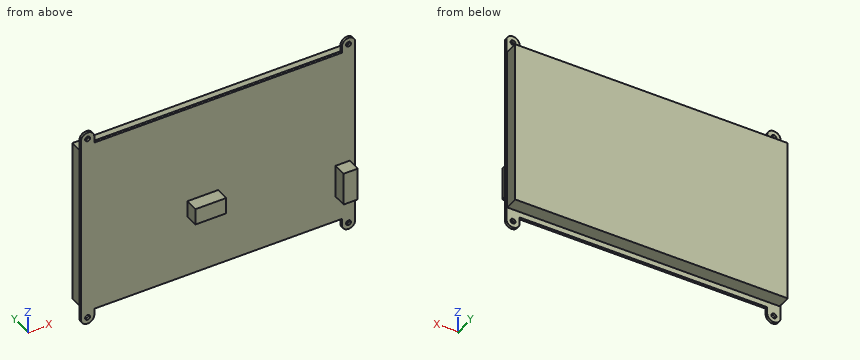
```python
from build123d import *

# Parameters (mm, degrees)
SKETCH1_R           = 1.5
BOSS_EXTRUDE1_DEPTH = 1.5
SKETCH2_W           = 8.49594542
SKETCH2_H           = 19.836738538
SKETCH2_W_2         = 18.514132699
SKETCH2_H_2         = 9.878260544
BOSS_EXTRUDE2_DEPTH = 8
SKETCH3_W           = 164
SKETCH3_H           = 100
BOSS_EXTRUDE3_DEPTH = 8


with BuildPart() as part:
    # Sketch1 → Boss-Extrude1 (new body)
    with BuildSketch(Plane(origin=(0, 0, 0), x_dir=(1, 0, 0), z_dir=(0, 1, 0))):
        with BuildLine():
            Line((-74.5, -53.5), (74.5, -53.5))
            Line((74.5, -53.5), (74.5, -57.5))
            ThreePointArc((74.5, -57.5), (78.5, -61.5), (82.5, -57.5))
            Line((82.5, -57.5), (82.5, -23.877612559))
            Line((82.5, -23.877612559), (82.5, 23.877612559))
            Line((82.5, 23.877612559), (82.5, 57.5))
            ThreePointArc((82.5, 57.5), (78.5, 61.5), (74.5, 57.5))
            Line((74.5, 57.5), (74.5, 53.5))
            Line((74.5, 53.5), (-74.5, 53.5))
            Line((-74.5, 53.5), (-74.5, 57.5))
            ThreePointArc((-74.5, 57.5), (-78.5, 61.5), (-82.5, 57.5))
            Line((-82.5, 57.5), (-82.5, 23.877612559))
            Line((-82.5, 23.877612559), (-82.5, -23.877612559))
            Line((-82.5, -23.877612559), (-82.5, -57.5))
            ThreePointArc((-82.5, -57.5), (-78.5, -61.5), (-74.5, -57.5))
            Line((-74.5, -57.5), (-74.5, -53.5))
        make_face()
        with Locations(Location((78.5, 57.5, 0), (0, 0, 270))):
            Circle(SKETCH1_R, mode=Mode.SUBTRACT)
        with Locations(Location((-78.5, 57.5, 0), (0, 0, 90))):
            Circle(SKETCH1_R, mode=Mode.SUBTRACT)
        with Locations(Location((78.5, -57.5, 0), (0, 0, 90))):
            Circle(SKETCH1_R, mode=Mode.SUBTRACT)
        with Locations(Location((-78.5, -57.5, 0), (0, 0, 270))):
            Circle(SKETCH1_R, mode=Mode.SUBTRACT)
    extrude(amount=BOSS_EXTRUDE1_DEPTH)

    # Sketch2 → Boss-Extrude2 (add)
    with BuildSketch(Plane.XZ):
        with Locations((74.922222093, -27.720858346)):
            Rectangle(SKETCH2_W, SKETCH2_H)
        with Locations((-9.25706635, -10.936720321)):
            Rectangle(SKETCH2_W_2, SKETCH2_H_2)
    extrude(amount=BOSS_EXTRUDE2_DEPTH)

    # Sketch3 → Boss-Extrude3 (add)
    with BuildSketch(Plane(origin=(0, 1.5, 0), x_dir=(1, 0, 0), z_dir=(0, 1, 0))):
        Rectangle(SKETCH3_W, SKETCH3_H)
    extrude(amount=BOSS_EXTRUDE3_DEPTH)


solid = part.part
```
The listing builds one solid part. Answer for the finished solid, in the listing's coordinates (mm). Round coordinates to 2 decimals unless told otherwise and drop trailing zeros. Order: outer loops, then holes, each group sorted by start corner. A loop starts at its lowest first (then second) coordinate and runs counter-clockwise, first axis right, second up. Notation, with made-up numbers: (47.25, -22.5) -> (88.25, -22.5) arc R16 ccw to (88.25, -9.5) -> close; hole circle Ø5 at (39, 86). An arc over 180 degrees is marked (long way). Answer as CSV lines item,"result". Start each with the question number.
(1) Flat-ended cylindrical pins translate along their axes: pin 1 Ø1 at (y, z) = (-2, 39) entering from +X (1 decimal); pin 2 Ø3 at (x, z) = (6, -47) entering from -Y; pin 3 Ø5 at (x, y) = (-42, 3) entering from +Z; pin 4 Ø5 at (x, z) = (-78.5, -57.5) entering from +Y. Find the tip coordinate at first contact, or state that the pin passes through.
(2) The part is cut by section B-B (x = -60). Determine the outline of the cut face in (y, z).
(3) The part is cut by section D-D (x = -7). Determine the outline of the cut face in (y, z), then the cut area to 3 significant figures.
(4) Find the intervals of material crossed by probe 1 along X at (y, z) = (1.1, -57.5); probe 2 along Z at (x, y) = (78.5, 1.1); probe 3 along Y at (x, z) = (-19.5, -3.5), in increasing order. Write a range as from..to.
(5) The part is cut by section C-C (z = 47). Determine the outline of the cut face in (x, y).
(6) The part is cut by section A-A (y = -2.5). Determine the outline of the cut face in (x, z).
Evaluation:
1,pin 1,"through"
1,pin 2,"y = 0"
1,pin 3,"z = 53.5"
1,pin 4,"y = 1.5"
2,outline,"(0, -53.5) -> (1.5, -53.5) -> (1.5, -50) -> (9.5, -50) -> (9.5, 50) -> (1.5, 50) -> (1.5, 53.5) -> (0, 53.5) -> close"
3,outline,"(-8, -15.88) -> (0, -15.88) -> (0, -53.5) -> (1.5, -53.5) -> (1.5, -50) -> (9.5, -50) -> (9.5, 50) -> (1.5, 50) -> (1.5, 53.5) -> (0, 53.5) -> (0, -6) -> (-8, -6) -> close"
3,area,"1,040 mm²"
4,probe 1,"-82.5..-80, -77..-74.5, 74.5..77, 80..82.5"
4,probe 2,"-61.5..-59, -56..56, 59..61.5"
4,probe 3,"0..9.5"
5,outline,"(-82.5, 0) -> (82.5, 0) -> (82.5, 1.5) -> (82, 1.5) -> (82, 9.5) -> (-82, 9.5) -> (-82, 1.5) -> (-82.5, 1.5) -> close"
6,outline,"(-18.51, -15.88) -> (0, -15.88) -> (0, -6) -> (-18.51, -6) -> close; (70.67, -37.64) -> (79.17, -37.64) -> (79.17, -17.8) -> (70.67, -17.8) -> close"
